from build123d import *

# Parameters (mm, degrees)
F1_DEPTH = 6


with BuildPart() as f1:
    # F0 (on Top) → F1 (new body)
    with BuildSketch(Plane.XY):
        with BuildLine():
            ThreePointArc((-2.050687, 23.429924), (-3.345865, 22.151504), (-5.01279, 21.421296))
            ThreePointArc((-5.01279, 21.421296), (0, -22), (5.01279, 21.421296))
            ThreePointArc((5.01279, 21.421296), (3.345865, 22.151504), (2.050687, 23.429924))
            ThreePointArc((2.050687, 23.429924), (0, 24.5), (-2.050687, 23.429924))
        make_face()
        with BuildLine():
            ThreePointArc((0, 20.5), (14.495689, 14.495689), (20.5, 0))
            ThreePointArc((20.5, 0), (-14.495689, -14.495689), (0, 20.5))
        make_face(mode=Mode.SUBTRACT)
        with BuildLine():
            ThreePointArc((1, 22), (0.707107, 21.292893), (0, 21))
            ThreePointArc((0, 21), (-0.707107, 22.707107), (1, 22))
        make_face(mode=Mode.SUBTRACT)
    extrude(amount=F1_DEPTH)


solid = f1.part
Design review of the part built by this model. Coordinates are the model's own, in mm. Round coordinates to 2 decimals unless told otherwise and drop trailing zeros. Write each loop counter-clockwise with the first axis right and the second up, starting at its lowest first coordinate (ties: lowest second). Pieces come first, ordered by that corner, then holes. Notation, with made-up numbers: (-3.5, 65.25) - (35.5, 65.25) arc R24 cw to (35.5, 100.25) - close; hole circle Ø8 at (46, -21). An arc over 180 degrees is marked (long way). Use a Markdown table: item, result. Add a question column.
1. Wall thickness on probe 1 along Y at (x, z) = (0, 4.5); probe 2 along X at (y, z) = (0.5, 0.5); probe 3 along Y at (x, z) = (-15.5, 0.7): over which ranges is each line inside the solid? List them lowest first.
2. We need section B-B (x = 9). State the section outline as (y, z) points, then the cut area to 3 significant figures.
3. Clearance check with flat-ended pins moving along their axes: pin 1 (1.5 mm diameter, centred on y = 5.5, z = 1.5, fed in from +X); pin 2 (1.2 mm diameter, centred on x = 0, y = 22, fed in from +Z); pin 3 (3 mm diameter, centred on x = 12.5, z = 4.5, fed in from -Y); pin 4 (1.5 mm diameter, centred on x = 13, z = 5, fed in from +Y). State where each tip first meets the part, or that it passes through.
4. We need section C-C (z = 2.5). State the section outline as (x, y) points.
5. We need section A-A (y = -15). State the section outline as (x, z) points.
Output:
| question | item | result |
|---|---|---|
| 1 | probe 1 | y = -22 to -20.5, 20.5 to 21, 23 to 24.5 |
| 1 | probe 2 | x = -21.99 to -20.49, 20.49 to 21.99 |
| 1 | probe 3 | y = -15.61 to -13.42, 13.42 to 15.61 |
| 2 | outline | (-20.07, 0) - (-18.42, 0) - (-18.42, 6) - (-20.07, 6) - close; (18.42, 0) - (20.07, 0) - (20.07, 6) - (18.42, 6) - close |
| 2 | area | 19.9 mm2 |
| 3 | pin 1 | stops at x = 21.48 |
| 3 | pin 2 | passes through |
| 3 | pin 3 | stops at y = -19.05 |
| 3 | pin 4 | stops at y = 18.27 |
| 4 | outline | (-5.01, 21.42) arc R22 ccw (long way) to (5.01, 21.42) arc R5 cw to (2.05, 23.43) arc R2.5 ccw to (-2.05, 23.43) arc R5 cw to start; hole circle Ø41 at (0, 0); hole circle Ø2 at (0, 22) |
| 5 | outline | (-16.09, 0) - (-13.97, 0) - (-13.97, 6) - (-16.09, 6) - close; (13.97, 0) - (16.09, 0) - (16.09, 6) - (13.97, 6) - close |
